Here's how the part is built. I have some questions about the finished solid (model axes, mm). Give positions to 0.01 mm unless a question says otherwise; leave off trailing zeros. Loops run counter-clockwise (first coordinate to the right, second up) from the corner with the lowest first, then second, coordinate; pieces in that order, holes last. Notation, with made-up numbers: M 82,-13 L 121,-13 A22 cw 121,3 Z; hole C -4,81.5 d9. An arc over 180 degrees is marked long. Answer as CSV lines item,"result". Start each with the question number.
Item 1: If I drill on line 1 along Y through (x, z) = (-1.5, 1.15); line 2 along Z through (x, y) = (-23.5, 0.35), over which ranges is the centre line in solid material (lowest first)? Write a range as from..to.
Item 2: I want a section at A-A on x = 14.5. List the corners of the cut face in (y, z) for me, plus the area to 3 significant figures.
Item 3: Will these pins go through, and if not, where does the flat tip stop? P1, Ø1.5, axis at x = -22, y = -1, coming from the -Z side; P2, Ø1, axis at x = 18, y = 1.5, coming from the +Z side.
from build123d import *

# Parameters (mm, degrees)
CHAMFER1_SIZE = 0.075


with BuildPart() as part:
    # Sketch2 → Revolve1 (revolve)
    with BuildSketch(Plane.XY):
        with BuildLine():
            Line((-30, 0), (30, 0))
            Line((30, 0), (30, 1))
            Line((30, 1), (21, 1))
            ThreePointArc((21, 1), (19.887839476, 1.264702229), (18.807410064, 1.638387373))
            ThreePointArc((18.807410064, 1.638387373), (17.891303231, 1.908764451), (16.940497485, 2))
            Line((16.940497485, 2), (-16.940497485, 2))
            ThreePointArc((-16.940497485, 2), (-17.891303231, 1.908764451), (-18.807410064, 1.638387373))
            ThreePointArc((-18.807410064, 1.638387373), (-19.887839476, 1.264702229), (-21, 1))
            Line((-21, 1), (-30, 1))
            Line((-30, 1), (-30, 0))
        make_face()
    revolve(axis=Axis((-30, 0, 0), (1, 0, 0)))

    # Chamfer1
    chamfer1_edges = [part.edges().sort_by_distance(p)[0] for p in [
        (30, -1, 0),
        (-30, -1, 0),
    ]]
    chamfer(chamfer1_edges, length=CHAMFER1_SIZE)


solid = part.part
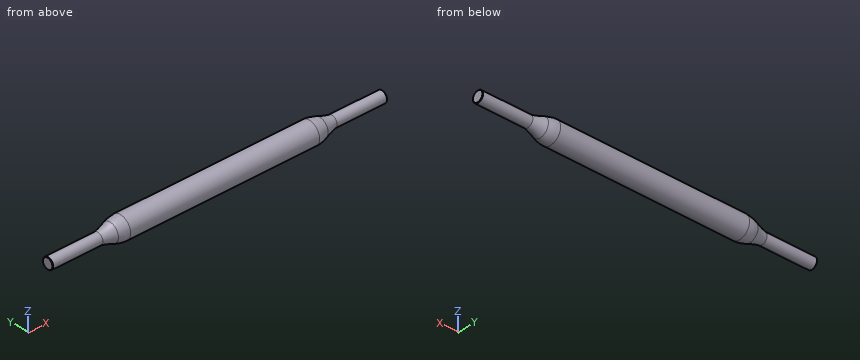
Result:
1,line 1,"-1.64..1.64"
1,line 2,"-0.94..0.94"
2,outline,"C 0,0 d4"
2,area,"12.6 mm^2"
3,P1,"z = -0.97"
3,P2,"z = 1.62"
